Check sheet for the drawn part. Datum: minimum x, y, z corner. Units: mm. Coordinates: 2 decimals unless noted, no trailing zeros. Order: outer loops, then holes, each group sorted by start corner. A loop starts at its lowest first (then second) coordinate and runs counter-clockwise, first axis right, second up. Notation, with made-up numbers: M -13.75,64.25 L 22.25,64.25 A14 cw 22.25,68.25 Z; hole C -34.5,-7.75 d3. An arc over 180 degrees is marked long. Return JSON: item names as keys, results as strings. Group by question number.
Q1. Section check C-C, the plane y = 32. Enter the section's corners in (x, z) (1 decimal), then the cut area to 3 significant figures.
Q2. Thickness scan on probe 1 along Z at (x, y) = (108.5, 5); probe 2 along X at (y, z) = (16, 35); probe 3 along Z at (x, y) = (43.5, 12) (1 decimal). Record the ranges inside material, lowest first.
Q3. Go/stop test with flat-tipped pins: pin 1 Ø4 at (x, y) = (111.5, 9) entering from +Z (1 decimal); pin 2 Ø6 at (y, z) = (34, 21) entering from +X; pin 3 Ø10 at (x, y) = (28.5, 33) entering from +Z. Record where each tip stops, or that it passes through.
Q4. Section check A-A, the plane z = 55. Enter the section's corners in (x, y) (1 decimal).
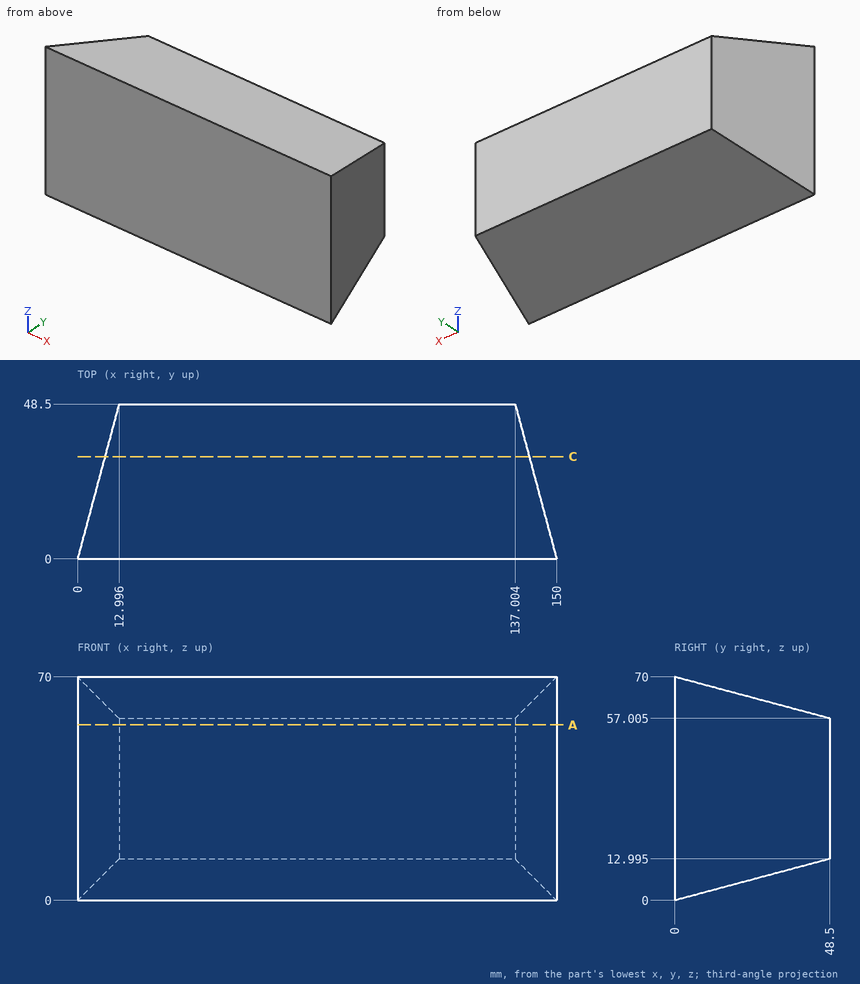
Numbers:
{
 "1": {"outline": "M 8.6,8.6 L 141.4,8.6 L 141.4,61.4 L 8.6,61.4 Z", "area": "7,020 mm2"},
 "2": {"probe 1": "z = 1.34 to 68.66", "probe 2": "x = 4.29 to 145.71", "probe 3": "z = 3.2 to 66.8"},
 "3": {"pin 1": "stops at z = 68.1", "pin 2": "stops at x = 141.69", "pin 3": "stops at z = 62.5"},
 "4": {"outline": "M 0,0 L 150,0 L 137,48.5 L 13,48.5 Z"}
}
